Design review of the part built by this model. Coordinates are the model's own, in mm. A direction names the side the tool comes from. Give positions to 0.01 mm unless a question says otherwise; leave off trailing zeros. Loops run counter-clockwise (first coordinate to the right, second up) from the corner with the lowest first, then second, coordinate; pieces in that order, holes last. Notation, with made-up numbers: M 29.5,36.25 L 69.5,36.25 A37 ccw 69.5,75.25 Z; hole C -0.5,-35.75 d9. An arc over 180 degrees is marked long. Use CSV: the item, a comma, the result in double quotes.
from build123d import *

# Parameters (mm, degrees)
F0_W      = 127
F0_H      = 63.5
F1_DEPTH  = 38.1
F2_W      = 76.2
F2_H      = 63.5
F3_DEPTH  = 20.32
F5_W      = 85.9366810061
F5_H      = 5.08
F6_DEPTH  = 34.798
F7_R      = 1.27
F12_R     = 2.54
F13_DEPTH = 30.48
F14_R     = 2.54
F15_DEPTH = 30.48
F17_W     = 2.54
F17_H     = 48.26
F18_DEPTH = 30.734
F19_W     = 2.54
F19_H     = 0.508
F20_DEPTH = 4.0894
F21_R     = 1.27
F22_DEPTH = 1.27
F23_W     = 2.54
F23_H     = 0.508
F24_DEPTH = 4.0894
F26_DEPTH = 1.27
F27_W     = 2.54
F27_H     = 0.508
F28_DEPTH = 4.0894
F29_R     = 1.27
F30_DEPTH = 1.27
F31_W     = 2.54
F31_H     = 0.508
F32_DEPTH = 4.0894
F33_R     = 1.27
F34_DEPTH = 1.27


with BuildPart() as f1:
    # F0 (on Top) → F1 (new body)
    with BuildSketch(Plane.XY):
        Rectangle(F0_W, F0_H)
    extrude(amount=F1_DEPTH)

    # F2 (on face) → F3 (join)
    with BuildSketch(Plane.XY.offset(38.1)):
        Rectangle(F2_W, F2_H)
    extrude(amount=F3_DEPTH)

    # F5 (on offset) → F6 (cut)
    with BuildSketch(Plane.XY.offset(74.676)):
        with Locations((1.5557501465, 24.8920014128)):
            Rectangle(F5_W, F5_H)
        with Locations((1.9367600847, 16.255996407)):
            Rectangle(F5_W, F5_H)
        with Locations((1.9685070086, 6.8579998174)):
            Rectangle(F5_W, F5_H)
        with Locations((2.1590034533, -1.8097495353)):
            Rectangle(F5_W, F5_H)
        with Locations((2.7622657884, -10.7949979296)):
            Rectangle(F5_W, F5_H)
        with Locations((2.2860284019, -18.9229918337)):
            Rectangle(F5_W, F5_H)
        with Locations((2.4130123723, -26.288997165)):
            Rectangle(F5_W, F5_H)
    extrude(amount=-F6_DEPTH, mode=Mode.SUBTRACT)

    # F7
    f7_edges = [f1.edges().sort_by_distance(p)[0] for p in [
        (-63.5, 0, 38.1),
        (-50.8, -31.75, 38.1),
        (-38.1, -6.302374, 58.42),
        (-38.1, -14.858995, 58.42),
        (-38.1, -30.289499, 58.42),
        (-38.1, -22.605994, 58.42),
        (-38.1, 11.556998, 58.42),
        (-38.1, 20.573999, 58.42),
        (-38.1, 29.591001, 58.42),
        (-38.1, 2.524125, 58.42),
        (-50.8, 31.75, 38.1),
        (63.5, 0, 38.1),
        (50.8, 31.75, 38.1),
        (50.8, -31.75, 38.1),
        (38.1, 2.524125, 58.42),
        (38.1, 11.556998, 58.42),
        (38.1, 20.573999, 58.42),
        (38.1, 29.591001, 58.42),
        (38.1, -6.302374, 58.42),
        (38.1, -14.858995, 58.42),
        (38.1, -22.605994, 58.42),
        (38.1, -30.289499, 58.42),
    ]]
    fillet(f7_edges, radius=F7_R)

    # F9 (on offset) → F11 (revolve, cut)
    with BuildSketch(Plane.XY.offset(69.342)):
        with BuildLine():
            Line((0, -27.1781864281), (0, 27.1781864281))
            ThreePointArc((0, 27.1781864281), (-27.1781864281, 0), (0, -27.1781864281))
        make_face()
    revolve(axis=Axis((0, 0.2222489566, 69.342), (0, -1, 0)), mode=Mode.SUBTRACT)

    # F12 (on face) → F13 (join)
    with BuildSketch(Plane.XY.offset(38.1)):
        with Locations((-57.15, 25.4)):
            Circle(F12_R)
        with Locations((-57.15, -25.4)):
            Circle(F12_R)
    extrude(amount=F13_DEPTH)

    # F14 (on face) → F15 (join)
    with BuildSketch(Plane.XY.offset(38.1)):
        with Locations((57.15, 25.4)):
            Circle(F14_R)
        with Locations((57.15, -25.4)):
            Circle(F14_R)
    extrude(amount=F15_DEPTH)

    # F17 (on offset) → F18 (cut)
    with BuildSketch(Plane.XY.offset(68.834)):
        with Locations((-57.15, 0)):
            Rectangle(F17_W, F17_H)
        with Locations((57.15, 0)):
            Rectangle(F17_W, F17_H)
    extrude(amount=-F18_DEPTH, mode=Mode.SUBTRACT)

    # F19 (on face) → F20 (join)
    with BuildSketch(Plane.XZ.offset(-24.13)):
        with Locations((-57.15, 68.326)):
            Rectangle(F19_W, F19_H)
    extrude(amount=F20_DEPTH)

    # F21 (on face) → F22 (join)
    with BuildSketch(Plane.XY.offset(68.58)):
        with Locations((-57.15, 21.3106)):
            Circle(F21_R)
    extrude(amount=F22_DEPTH)

    # F23 (on face) → F24 (join)
    with BuildSketch(Plane(origin=(0, -24.13, 0), x_dir=(-1, 0, 0), z_dir=(0, 1, 0))):
        with Locations((57.15, 68.326)):
            Rectangle(F23_W, F23_H)
    extrude(amount=F24_DEPTH)

    # F25 (on face) → F26 (join)
    with BuildSketch(Plane.XY.offset(68.58)):
        with BuildLine():
            ThreePointArc((-58.42, -21.3106), (-57.15, -22.5806), (-55.88, -21.3106))
            ThreePointArc((-55.88, -21.3106), (-56.2519743879, -20.4125743879), (-57.15, -20.0406))
            ThreePointArc((-57.15, -20.0406), (-58.0480256121, -20.4125743879), (-58.42, -21.3106))
        make_face()
    extrude(amount=F26_DEPTH)

    # F27 (on face) → F28 (join)
    with BuildSketch(Plane.XZ.offset(-24.13)):
        with Locations((57.15, 68.326)):
            Rectangle(F27_W, F27_H)
    extrude(amount=F28_DEPTH)

    # F29 (on face) → F30 (join)
    with BuildSketch(Plane.XY.offset(68.58)):
        with Locations((57.15, 21.3106)):
            Circle(F29_R)
    extrude(amount=F30_DEPTH)

    # F31 (on face) → F32 (join)
    with BuildSketch(Plane(origin=(0, -24.13, 0), x_dir=(-1, 0, 0), z_dir=(0, 1, 0))):
        with Locations((-57.15, 68.326)):
            Rectangle(F31_W, F31_H)
    extrude(amount=F32_DEPTH)

    # F33 (on face) → F34 (join)
    with BuildSketch(Plane.XY.offset(68.58)):
        with Locations((57.15, -21.3106)):
            Circle(F33_R)
    extrude(amount=F34_DEPTH)


solid = f1.part
(1) The part is to be moulded in two halves that separate along X. For faces 6 (the flat face through (57, 21, 69.85)), 7 (the cylindrical face through (-57.06, 27.94, 53.13)), say which applies: released by +X, released by -X, zero draft, split by the parting line, or undercut.
A:
face 6,"zero draft"
face 7,"undercut"
(2) Clearance check with flat-ended pins moving along their axes: P1, Ø2, axis at y = -8.5, z = 43, coming from the +X side; P2, Ø5, axis at x = -50.5, z = 60.5, coming from the +Y side; P3, Ø5, axis at x = 38, y = 16.5, coming from the +Z side; P4, Ø1.5, axis at x = -17, y = -19, coming from the +Z side. State where each tip first meets the part, or that it passes through.
A:
P1,"x = 38.1"
P2,"through"
P3,"z = 58.41"
P4,"z = 39.88"
(3) We need section A-A on y = 25.4. State the section outline as (x, z) points.
A:
outline,"M -63.5,0 L 63.5,0 L 63.5,36.83 A1.27 ccw 62.23,38.1 L 59.69,38.1 L 59.69,68.58 L 54.61,68.58 L 54.61,38.1 L 38.1,38.1 L 38.1,39.88 L -38.1,39.88 L -38.1,38.1 L -54.61,38.1 L -54.61,68.58 L -59.69,68.58 L -59.69,38.1 L -62.23,38.1 A1.27 ccw -63.5,36.83 Z"
(4) Wall thickness on line 1 along X through (y, z) = (-24, 66); line 2 along Z through (x, y) = (5, -19.5); line 3 along Y through (x, z) = (-47.5, 37): over which ranges is each line inside the solid? List them lowest first. Write a range as [from, to].
A:
line 1,"[-59.27, -58.42], [-55.88, -55.03], [55.03, 55.88], [58.42, 59.27]"
line 2,"[0, 39.88]"
line 3,"[-31.74, 31.74]"
(5) Machinability: for faces 1 (the flat face through (-1, 0, 0)), 2 (the flat face through (-1, 9.398, 43)), 3 (the cylindrical face through (57.06, -27.94, 53.13)), 4 (the flat face through (-57, -21, 69.85)), 5 (the flat face through (57, -24.13, 53)), which of the approach directions +Z, -Z, +X, -X, +Y, -Y give a long, thin tool a straight path to every point of the face, cutting with its end or side? Answer none if there is none.
A:
face 1,"-Z, +X, -X, +Y, -Y"
face 2,"+Z, +X, -X"
face 3,"+Z"
face 4,"+Z, +X, -X, +Y, -Y"
face 5,"none"
(6) We need section C-C on z = 54. Count the separate pieces of the cut face and the enclosed holes in it, then the cut area to 3 significant figures.
A:
separate pieces,"17"
enclosed holes,"0"
area,"1,530 mm²"
(7) We need section D-D on y = 6. State the section outline as (x, z) points, then the cut area to 3 significant figures.
A:
outline,"M -63.5,0 L 63.5,0 L 63.5,36.83 A1.27 ccw 62.23,38.1 L 38.1,38.1 L 38.1,39.88 L -38.1,39.88 L -38.1,38.1 L -62.23,38.1 A1.27 ccw -63.5,36.83 Z"
area,"4,970 mm²"
